Input: part model. Units: mm. Frame: model coordinates. Face numbers are marked on the shaded views. A direction names the side the tool comes from. Give positions to 0.01 mm unless a question says otherwise; leave off trailing zeros. Order: outer loops, then holes, each group sorted by start corner. A loop starts at its lowest first (then second) coordinate and runs counter-clockwise, first axis right, second up.
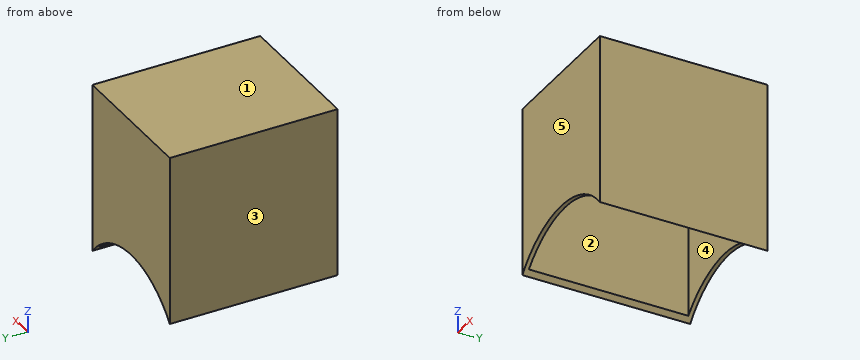
```python
from build123d import *

# Parameters (mm, degrees)
F1_DEPTH = 101.6
F2_T     = -2.54


with BuildPart() as f1:
    # F0 (on Front) → F1 (new body)
    with BuildSketch(Plane.XZ):
        with BuildLine():
            Line((39.729103, 49.523432), (-44.695243, 49.523432))
            Line((-44.695243, 49.523432), (-44.695243, -53.661879))
            ThreePointArc((-44.695243, -53.661879), (-2.48307, -33.383303), (39.729103, -53.661879))
            Line((39.729103, -53.661879), (39.729103, 49.523432))
        make_face()
    extrude(amount=F1_DEPTH)

    # F2
    f2_openings = [f1.faces().sort_by_distance(p)[0] for p in [
        (-2.48307, -50.8, -33.383303),
    ]]
    offset(amount=F2_T, openings=f2_openings)


solid = f1.part
```
1) Line query: probe 1 along Y at (x, z) = (15.5, -9); probe 2 along X at (y, z) = (-6.5, 15.5); probe 3 along Z at (x, y) = (-7.5, -82.5). Output: solid intervals per line, ascending.
2) Reachability of the marked faces 4 and 5 from +Z, -Z, +X, -X, +Y, -Y: full face, straight path, thin tool, end or side. Return the list, or none.
3) Cut plane B-B (x = -2.5). Return the cut outline in (y, z), then the cut area to 3 significant figures.
4) Cut plane D-D (z = -45). Return the cut outline in (x, y), then the cut area to 3 significant figures.
5) Pull-direction query (X, two-part tool) for the marked faces 1, 2 and 3; classes: pulls with the +X half, pulls with the -X half, needs draft (parallel to the pull), parting line crosses it, or undercut.
6) Cut plane A-A (z = 0). Return the cut outline in (x, y), then the cut area to 3 significant figures.
7) First-contact query: P1, Ø3, axis at x = -23, y = -27, coming from the -Z side. Flat tip, straight axial feed; report the tip coordinate or a pass-through.
8) Cut plane C-C (y = -49.5). Return the cut outline in (x, z), then the cut area to 3 significant figures.
Geometry says:
1. probe 1: y = -101.6 to -99.06, -2.54 to 0
1. probe 2: x = -44.7 to -42.16, 37.19 to 39.73
1. probe 3: z = 46.98 to 49.52
2. face 4: -Z
2. face 5: +Z, -Z, +X, -X, -Y
3. outline: (-101.6, -33.38) - (-99.06, -33.38) - (-99.06, 46.98) - (-2.54, 46.98) - (-2.54, -33.38) - (0, -33.38) - (0, 49.52) - (-101.6, 49.52) - close
3. area: 666 mm2
4. outline: (-44.7, -101.6) - (-35.97, -101.6) - (-35.97, -99.06) - (-42.16, -99.06) - (-42.16, -2.54) - (-35.97, -2.54) - (-35.97, 0) - (-44.7, 0) - close; (31, -101.6) - (39.73, -101.6) - (39.73, 0) - (31, 0) - (31, -2.54) - (37.19, -2.54) - (37.19, -99.06) - (31, -99.06) - close
4. area: 579 mm2
5. face 1: needs draft
5. face 2: undercut
5. face 3: pulls with the -X half
6. outline: (-44.7, -101.6) - (39.73, -101.6) - (39.73, 0) - (-44.7, 0) - close; hole (-42.16, -99.06) - (37.19, -99.06) - (37.19, -2.54) - (-42.16, -2.54) - close
6. area: 919 mm2
7. P1: stops at z = 46.98
8. outline: (-44.7, -53.66) arc R54.07 cw to (-42.16, -50.71) - (-42.16, 46.98) - (37.19, 46.98) - (37.19, -50.71) arc R54.07 cw to (39.73, -53.66) - (39.73, 49.52) - (-44.7, 49.52) - close
8. area: 718 mm2
